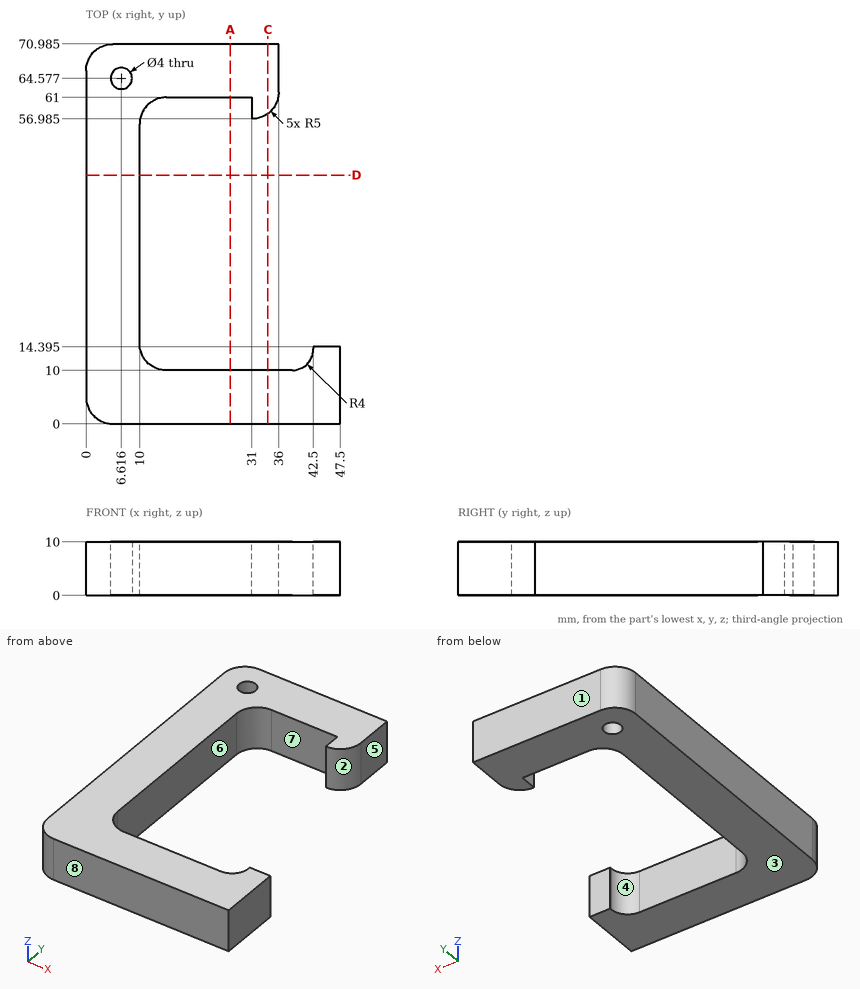
Here's the drawing with two shaded views (mm, measured from the low corner). I have some questions. A direction names the side the tool comes from. Coordinates: 2 decimals unless noted, no trailing zeros. Order: outer loops, then holes, each group sorted by start corner. A loop starts at its lowest first (then second) coordinate and runs counter-clockwise, first axis right, second up. Notation, with made-up numbers: (-8.75, 5) - (24.25, 5) arc R18 ccw to (24.25, 9) - close; hole circle Ø5 at (-24, -3). An arc over 180 degrees is marked (long way). Answer in a Markdown table with one row per item.
1. If we mould it in two halves opening along Y, with no side actions, what happens to the marked faces 1, 2 and 3? For each: pulls with the +Y half, pulls with the -Y half, needs draft (parallel to the pull), parting line crosses it, or undercut.
Reply:
| item | result |
|---|---|
| face 1 | pulls with the +Y half |
| face 2 | undercut |
| face 3 | needs draft |
2. Suppose I cut it at D-D (y = 46.5). Please give me the cut outline in (x, z).
Reply:
| item | result |
|---|---|
| outline | (0, 0) - (10, 0) - (10, 10) - (0, 10) - close |
3. Suppose I cut it at A-A (x = 27). Please give me the cut outline in (y, z) (1 decimal), and give its area (3 significant figures).
Reply:
| item | result |
|---|---|
| outline | (0, 0) - (10, 0) - (10, 10) - (0, 10) - close; (61, 0) - (71, 0) - (71, 10) - (61, 10) - close |
| area | 200 mm^2 |
4. For the marked faces 4, 5, 6, 7 and 8, which set-ups out of +Z, -Z, +X, -X, +Y, -Y let a thin tool reach every point of the face, with its end or its side?
Reply:
| item | result |
|---|---|
| face 4 | +Z, -Z, +Y |
| face 5 | +Z, -Z, +X, +Y |
| face 6 | +Z, -Z, +X |
| face 7 | +Z, -Z |
| face 8 | +Z, -Z, +X, -X, -Y |
5. If I drill on line 1 along Y through (x, z) = (25.5, 5.75) (1 decimal); line 2 along X through (y, z) = (17.5, 2.5); line 3 along X through (y, z) = (60.5, 5.5) (1 decimal), over which ranges is the centre line in solid material (lowest first)?
Reply:
| item | result |
|---|---|
| line 1 | y = 0 to 10, 61 to 71 |
| line 2 | x = 0 to 10 |
| line 3 | x = 0 to 12.8, 31 to 35.8 |
6. Suppose I cut it at C-C (x = 34). Please give me the cut outline in (y, z) (1 decimal).
Reply:
| item | result |
|---|---|
| outline | (0, 0) - (10, 0) - (10, 10) - (0, 10) - close; (58, 0) - (71, 0) - (71, 10) - (58, 10) - close |
7. For pin 1 (1.5 mm diameter, centred on x = 45.5, z = 5, fed in from +Y) (1 decimal); pin 2 (2 mm diameter, centred on y = 43.5, z = 3.5, fed in from +X), each with a flat end and sliding along its axis, tell me the tip position at first contact or that it passes through.
Reply:
| item | result |
|---|---|
| pin 1 | stops at y = 14.4 |
| pin 2 | stops at x = 10 |
